Geometry check sheet. Reference: the model listing, model coordinates, mm. A direction names the side the tool comes from. Round coordinates to 2 decimals unless told otherwise and drop trailing zeros. Loops run counter-clockwise (first coordinate to the right, second up) from the corner with the lowest first, then second, coordinate; pieces in that order, holes last. Notation, with made-up numbers: (-18.75, 34) - (-6.75, 34) arc R16 cw to (-6.75, 51) - close; hole circle Ø1 at (71, 7). An arc over 180 degrees is marked (long way). Write item = value, one per line.
```python
from build123d import *

# Parameters (mm, degrees)
SKETCH_2_W               = 140
SKETCH_2_H               = 140
EXTRUDE_1_DEPTH          = 500
FILLET_1_R               = 70
FILLET_2_R               = 70
SKETCH_5_W               = 100
SKETCH_5_H               = 141.285409295
CUT_EXTRUDE_2_DEPTH      = 300
CUT_EXTRUDE_START        = -20
SKETCH_6_R               = 80
CUT_EXTRUDE_3_DEPTH      = 100
SKETCH_8_W               = 100
SKETCH_8_H               = 420
CUT_EXTRUDE_4_DEPTH      = 188
CUT_EXTRUDE_6_DEPTH      = 185
SKETCH_10_W              = 46
SKETCH_10_H              = 24.912851684
CUT_EXTRUDE_7_DEPTH      = 185
CUT_EXTRUDE_9_DEPTH      = 192
CUT_EXTRUDE_9_DEPTH_BACK = 192
SKETCH_12_W              = 70.971879984
SKETCH_12_H              = 535.265340004
SKETCH_13_R              = 5
CUT_EXTRUDE_10_DEPTH     = 192
SKETCH_15_R              = 29.5
CUT_EXTRUDE_11_DEPTH     = 10
SKETCH_17_R              = 2
CUT_EXTRUDE_12_DEPTH     = 10
SKETCH_18_R              = 29.5
CUT_EXTRUDE_14_DEPTH     = 10
SKETCH_20_R              = 2
CUT_EXTRUDE_15_DEPTH     = 10


with BuildPart() as part:
    # 草图2 → 凸台-拉伸1 (new body)
    with BuildSketch(Plane(origin=(0, 0, 0), x_dir=(1, 0, 0), z_dir=(0, 1, 0))):
        Rectangle(SKETCH_2_W, SKETCH_2_H)
    extrude(amount=EXTRUDE_1_DEPTH)

    # 圆角1
    fillet_1_edges = [part.edges().sort_by_distance(p)[0] for p in [
        (0, 500, -70),
        (0, 500, 70),
    ]]
    fillet(fillet_1_edges, radius=FILLET_1_R - 0.0001)  # a hair under: the kernel refuses the full size

    # 圆角2
    fillet_2_edges = [part.edges().sort_by_distance(p)[0] for p in [
        (0, 0, 70),
        (0, 0, -70),
    ]]
    fillet(fillet_2_edges, radius=FILLET_2_R - 0.0001)  # a hair under: the kernel refuses the full size

    # 草图5 → 切除-拉伸2 (cut)
    with BuildSketch(Plane.XY.offset(70)):
        with Locations((0, 430.642704648)):
            Rectangle(SKETCH_5_W, SKETCH_5_H)
    extrude(amount=-CUT_EXTRUDE_2_DEPTH, mode=Mode.SUBTRACT)

    # 草图6 → 切除-拉伸3 (cut)
    with BuildSketch(Plane(origin=(70, 0, 0), x_dir=(0, 0, -1), z_dir=(1, 0, 0)).offset(CUT_EXTRUDE_START)):
        with Locations((0, 430)):
            Circle(SKETCH_6_R)
        with Locations((0, 70)):
            Circle(SKETCH_6_R)
    extrude(amount=-CUT_EXTRUDE_3_DEPTH, mode=Mode.SUBTRACT)

    # 草图8 → 切除-拉伸4 (cut)
    with BuildSketch(Plane.XY.offset(70)):
        with Locations((0, 210)):
            Rectangle(SKETCH_8_W, SKETCH_8_H)
    extrude(amount=-CUT_EXTRUDE_4_DEPTH, mode=Mode.SUBTRACT)


with BuildPart() as cut_extrude_4_piece_1:
    # of the separate pieces the step leaves, piece 1, a body of its own (cut_extrude_4_pieces)
    add(part.part.solids().sort_by_distance((-70, 69.9999, 70))[0])


with BuildPart() as cut_extrude_4_piece_2:
    # of the separate pieces the step leaves, piece 2, a body of its own (cut_extrude_4_pieces)
    add(part.part.solids().sort_by_distance((50, 69.9999, 70))[0])


with BuildPart() as cut_extrude_6_tool:
    # 草图9 → 切除-拉伸6 (new body)
    with BuildSketch(Plane.ZY.offset(70)):
        with BuildLine():
            Line((-70, 430), (-70, 70))
            ThreePointArc((-70, 70), (-63.981049548, 98.3976284), (-46.959277178, 121.911716278))
            Line((-46.959277178, 121.911716278), (-46.959277178, 378.088283722))
            ThreePointArc((-46.959277178, 378.088283722), (-63.981049548, 401.6023716), (-70, 430))
        make_face()
        with BuildLine():
            Line((46.959277178, 378.088283722), (46.959277178, 121.911716278))
            ThreePointArc((46.959277178, 121.911716278), (63.981049548, 98.3976284), (70, 70))
            Line((70, 70), (70, 430))
            ThreePointArc((70, 430), (63.981049548, 401.6023716), (46.959277178, 378.088283722))
        make_face()
    extrude(amount=-CUT_EXTRUDE_6_DEPTH)


with BuildPart() as cut_extrude_4_piece_1_1:
    add(cut_extrude_4_piece_1.part)

    # 切除-拉伸6: cut by cut_extrude_6_tool
    add(cut_extrude_6_tool.part, mode=Mode.SUBTRACT)


with BuildPart() as cut_extrude_4_piece_2_1:
    add(cut_extrude_4_piece_2.part)

    # 切除-拉伸6: cut by cut_extrude_6_tool
    add(cut_extrude_6_tool.part, mode=Mode.SUBTRACT)


with BuildPart() as cut_extrude_7_tool:
    # 草图10 → 切除-拉伸7 (new body)
    with BuildSketch(Plane(origin=(70, 0, 0), x_dir=(0, 0, -1), z_dir=(1, 0, 0))):
        with Locations((0, 301.446288317)):
            Rectangle(SKETCH_10_W, SKETCH_10_H)
        with Locations((0, 351.446288317)):
            Rectangle(SKETCH_10_W, SKETCH_10_H)
        with Locations((0, 251.446288317)):
            Rectangle(SKETCH_10_W, SKETCH_10_H)
        with Locations((0, 201.446288317)):
            Rectangle(SKETCH_10_W, SKETCH_10_H)
        with Locations((0, 151.446288317)):
            Rectangle(SKETCH_10_W, SKETCH_10_H)
    extrude(amount=-CUT_EXTRUDE_7_DEPTH)


with BuildPart() as cut_extrude_4_piece_1_2:
    add(cut_extrude_4_piece_1_1.part)

    # 切除-拉伸7: cut by cut_extrude_7_tool
    add(cut_extrude_7_tool.part, mode=Mode.SUBTRACT)

    # 草图13 → 切除-拉伸10 (cut)
    with BuildSketch(Plane.ZY.offset(70)):
        with Locations((-33.507435555, 326.527789487)):
            Circle(SKETCH_13_R)
        with Locations((34.492564445, 326.527789487)):
            Circle(SKETCH_13_R)
        with Locations((-33.507435555, 276.527789487)):
            Circle(SKETCH_13_R)
        with Locations((-33.507435555, 226.527789487)):
            Circle(SKETCH_13_R)
        with Locations((-33.507435555, 176.527789487)):
            Circle(SKETCH_13_R)
        with Locations((34.492564445, 276.527789487)):
            Circle(SKETCH_13_R)
        with Locations((34.492564445, 226.527789487)):
            Circle(SKETCH_13_R)
        with Locations((34.492564445, 176.527789487)):
            Circle(SKETCH_13_R)
    extrude(amount=-CUT_EXTRUDE_10_DEPTH, mode=Mode.SUBTRACT)

    # 草图15 → 切除-拉伸11 (cut)
    with BuildSketch(Plane.ZY.offset(70)):
        with Locations((0, 70)):
            Circle(SKETCH_15_R)
    extrude(amount=-CUT_EXTRUDE_11_DEPTH, mode=Mode.SUBTRACT)

    # 草图17 → 切除-拉伸12 (cut)
    with BuildSketch(Plane.ZY.offset(60)):
        with Locations((-9.287970724, 84.53602765)):
            Circle(SKETCH_17_R)
        with Locations((7.944583853, 85.311632421)):
            Circle(SKETCH_17_R)
        with Locations((17.232554577, 70.775604771)):
            Circle(SKETCH_17_R)
        with Locations((9.287970724, 55.46397235)):
            Circle(SKETCH_17_R)
        with Locations((-7.944583853, 54.688367579)):
            Circle(SKETCH_17_R)
        with Locations((-17.232554577, 69.224395229)):
            Circle(SKETCH_17_R)
    extrude(amount=-CUT_EXTRUDE_12_DEPTH, mode=Mode.SUBTRACT)

    # 草图18 → 切除-拉伸14 (cut)
    with BuildSketch(Plane.ZY.offset(70)):
        with Locations((0, 430)):
            Circle(SKETCH_18_R)
    extrude(amount=-CUT_EXTRUDE_14_DEPTH, mode=Mode.SUBTRACT)

    # 草图20 → 切除-拉伸15 (cut)
    with BuildSketch(Plane.ZY.offset(60)):
        with Locations((-0.697918411, 449.237344149)):
            Circle(SKETCH_20_R)
        with Locations((16.311069529, 440.223087148)):
            Circle(SKETCH_20_R)
        with Locations((17.00898794, 420.985742999)):
            Circle(SKETCH_20_R)
        with Locations((0.697918411, 410.762655851)):
            Circle(SKETCH_20_R)
        with Locations((-16.311069529, 419.776912852)):
            Circle(SKETCH_20_R)
        with Locations((-17.00898794, 439.014257001)):
            Circle(SKETCH_20_R)
    extrude(amount=-CUT_EXTRUDE_15_DEPTH, mode=Mode.SUBTRACT)


with BuildPart() as cut_extrude_4_piece_2_2:
    add(cut_extrude_4_piece_2_1.part)

    # 切除-拉伸7: cut by cut_extrude_7_tool
    add(cut_extrude_7_tool.part, mode=Mode.SUBTRACT)

    # 草图12 → 切除-拉伸9 (cut, two sides: drawn at the far end of the back side and taken through both)
    with BuildSketch(Plane(origin=(0, 0, -46.959277178), x_dir=(-1, 0, 0), z_dir=(0, 0, -1)).offset(-CUT_EXTRUDE_9_DEPTH_BACK)):
        with Locations((-52.025627734, 250)):
            Rectangle(SKETCH_12_W, SKETCH_12_H)
    extrude(amount=CUT_EXTRUDE_9_DEPTH + CUT_EXTRUDE_9_DEPTH_BACK, mode=Mode.SUBTRACT)


solid = cut_extrude_4_piece_1_2.part
```
(1) Set-up check for faces 1 (the cylindrical face through (-59.86, 478.95, 50.04)), 2 (the flat face through (-60, 201, -23)), 3 (the flat face through (-60, 430, 0)): record each of +Z, -Z, +X, -X, +Y, -Y from which the full face is reachable in a straight line by a thin tool's end or side.
Answers follow:
face_1 = +Z, +X, -X, +Y
face_2 = +X, -X
face_3 = -X
(2) Section check B-B (y = 464.5). Enter the section's corners in (x, z), then the cut area to 3 significant figures.
Answers follow:
outline = (-70, -60.91) - (-50, -60.91) - (-50, 60.91) - (-70, 60.91) - close
area = 2,440 mm²
(3) Gauge pin test, flat ends, axial feed: pin 1 (10 mm diameter, centred on x = -55, y = 58, fed in from -Z); pin 2 (8 mm diameter, centred on x = -61.5, y = 389.5, fed in from +Z); pin 3 (6 mm diameter, centred on x = -57, y = 206.5, fed in from +Z). Record the tip position at first contact, or that the pin passes through.
Answers follow:
pin_1 = -69.65
pin_2 = 59.73
pin_3 = 46.96
(4) Section check A-A (y = 201). Enter the section's corners in (x, z).
Answers follow:
outline = (-70, -46.96) - (-50, -46.96) - (-50, -23) - (-70, -23) - close; (-70, 23) - (-50, 23) - (-50, 46.96) - (-70, 46.96) - close
(5) Mould release check, pull along Y, two halves, no side actions. Record for faces 4 (the cylindrical face through (-59.86, 19.96, -48.95)), 5 (the flat face through (-60, 351, 23)), 6 (the cylindrical face through (-60.14, 231.485, 33.842)), 7 (the cylindrical face through (-59.86, 478.95, -50.04)): pulls with the +Y half, pulls with the -Y half, needs draft (parallel to the pull), parting line crosses it, or undercut.
Answers follow:
face_4 = pulls with the -Y half
face_5 = undercut
face_6 = undercut
face_7 = pulls with the +Y half
(6) Scan lines: L1, parallel to Z at x = -51, y = 308; L2, parallel to Y at x = -58, z = 63.5; L3, parallel to Y at x = -62.75, z = -23.5. Record each from-to range of solid material in increasing order. Write a range as [from, to].
Answers follow:
L1 = [-46.96, -23], [23, 46.96]
L2 = [40.54, 99.46], [400.54, 459.46]
L3 = [4.06, 52.17], [87.83, 412.17], [447.83, 495.94]
